```python
from build123d import *

# Parameters (mm, degrees)
BOSS_EXTRUDE1_DEPTH = 1.524
CUT_EXTRUDE1_DEPTH  = 1.524


with BuildPart() as part:
    # Sketch1 → Boss-Extrude1 (new body)
    with BuildSketch(Plane.XY):
        with BuildLine():
            Line((-65.62844389, -1.524), (-63.025670989, -1.524))
            Line((-63.025670989, -1.524), (-63.822514801, -3.597982164))
            Line((-63.822514801, -3.597982164), (-66.364740688, -5.02874479))
            Line((-66.364740688, -5.02874479), (-72.970412181, -5.02874479))
            ThreePointArc((-72.970412181, -5.02874479), (-73.780479042, -4.88253576), (-74.589728748, -4.731869528))
            Line((-74.589728748, -4.731869528), (-75.073084302, -7.372952412))
            Line((-75.073084302, -7.372952412), (-75.51502387, -4.553940069))
            ThreePointArc((-75.51502387, -4.553940069), (-79.267617574, -3.769993691), (-82.998880802, -2.890103837))
            Line((-82.998880802, -2.890103837), (-83.662208167, -4.580640418))
            Line((-83.662208167, -4.580640418), (-83.9742265, -2.643374593))
            ThreePointArc((-83.9742265, -2.643374593), (-87.594512539, -1.666053196), (-91.189152721, -0.598256357))
            Line((-91.189152721, -0.598256357), (-91.929187087, -1.873078309))
            Line((-91.929187087, -1.873078309), (-92.192549363, -0.282576404))
            ThreePointArc((-92.192549363, -0.282576404), (-94.43829357, 0.452244536), (-96.672145794, 1.2224608))
            ThreePointArc((-96.672145794, 1.2224608), (-98.79856677, 2.920982901), (-100.989304929, 4.535699537))
            Line((-100.989304929, 4.535699537), (-102.141504416, 2.851715672))
            Line((-102.141504416, 2.851715672), (-101.830844258, 5.121924515))
            ThreePointArc((-101.830844258, 5.121924515), (-105.503835902, 7.476274523), (-109.316148256, 9.597619873))
            Line((-109.316148256, 9.597619873), (-110.95226101, 7.891468444))
            Line((-110.95226101, 7.891468444), (-110.319639872, 10.105642428))
            ThreePointArc((-110.319639872, 10.105642428), (-116.815196671, 12.929470472), (-123.562513889, 15.083530197))
            ThreePointArc((-123.562513889, 15.083530197), (-123.779823463, 15.177511529), (-123.959746364, 15.331406595))
            ThreePointArc((-123.959746364, 15.331406595), (-123.949496649, 18.088692586), (-121.216404531, 18.453300008))
            ThreePointArc((-121.216404531, 18.453300008), (-119.99831308, 17.594979685), (-118.73086738, 16.811371391))
            Line((-118.73086738, 16.811371391), (-117.11063531, 18.184449417))
            Line((-117.11063531, 18.184449417), (-117.859531811, 16.331247904))
            ThreePointArc((-117.859531811, 16.331247904), (-113.341616748, 14.499894981), (-108.552725398, 13.587793188))
            ThreePointArc((-108.552725398, 13.587793188), (-107.803028846, 13.376700844), (-107.057015293, 13.152940531))
            Line((-107.057015293, 13.152940531), (-106.609325514, 15.13772615))
            Line((-106.609325514, 15.13772615), (-106.122626057, 12.853069881))
            ThreePointArc((-106.122626057, 12.853069881), (-103.421109493, 11.859213859), (-100.787074077, 10.698266414))
            Line((-100.787074077, 10.698266414), (-99.448684771, 12.381094003))
            Line((-99.448684771, 12.381094003), (-100.023702083, 10.324148845))
            ThreePointArc((-100.023702083, 10.324148845), (-96.831167643, 8.560951785), (-93.788416789, 6.550278449))
            Line((-93.788416789, 6.550278449), (-92.677002467, 8.368956431))
            Line((-92.677002467, 8.368956431), (-92.959454339, 5.939754488))
            ThreePointArc((-92.959454339, 5.939754488), (-91.397772197, 4.708540381), (-89.890787426, 3.410951775))
            ThreePointArc((-89.890787426, 3.410951775), (-84.591869737, 0.643036614), (-78.809267625, 2.160071819))
            ThreePointArc((-78.809267625, 2.160071819), (-77.644578081, 2.700645179), (-76.424081928, 3.09953167))
            Line((-76.424081928, 3.09953167), (-76.558408494, 5.228958142))
            Line((-76.558408494, 5.228958142), (-75.149258413, 3.353285973))
            ThreePointArc((-75.149258413, 3.353285973), (-73.933139466, 3.450839152), (-72.713766302, 3.410951775))
            Line((-72.713766302, 3.410951775), (-66.233949818, 3.410951775))
            Line((-66.233949818, 3.410951775), (-63.424092895, 1.94149826))
            Line((-63.424092895, 1.94149826), (-63.025670989, 0))
            Line((-63.025670989, 0), (-65.62844389, 0))
            Line((-65.62844389, 0), (-65.62844389, -1.524))
        make_face()
    extrude(amount=BOSS_EXTRUDE1_DEPTH)

    # Sketch2 → Cut-Extrude1 (cut)
    with BuildSketch(Plane.XY.offset(1.524)):
        Polygon((-126.267748699, 16.679917712), (-121.799652461, 15.482694933), (-121.405212236, 16.954765892), (-125.873308475, 18.151988671), align=None)
    extrude(amount=-CUT_EXTRUDE1_DEPTH, mode=Mode.SUBTRACT)


solid = part.part
```
For this review, take the finished solid that the model builds, in its own axes (mm). A direction names the side the tool comes from. Round coordinates to 2 decimals unless told otherwise and drop trailing zeros. Write each loop counter-clockwise with the first axis right and the second up, starting at its lowest first coordinate (ties: lowest second). Pieces come first, ordered by that corner, then holes. Notation, with made-up numbers: (48.25, 28.25) - (52.25, 28.25) arc R15 ccw to (52.25, 54.25) - close; hole circle Ø9 at (30, -16.5). An arc over 180 degrees is marked (long way). Answer as a JSON object with one key per item and string values.
1. We need section C-C on x = -114.5. Give the boundary of the cut face in (y, z).
Response values:
{"outline": "(12.01, 0) - (14.87, 0) - (14.87, 1.52) - (12.01, 1.52) - close"}
2. We need section A-A on y = 4. Give the boundary of the cut face in (x, z), then the cut area to 3 significant figures.
Response values:
{"outline": "(-101.98, 0) - (-101.36, 0) - (-101.36, 1.52) - (-101.98, 1.52) - close; (-100.24, 0) - (-90.56, 0) - (-90.56, 1.52) - (-100.24, 1.52) - close; (-76.48, 0) - (-75.64, 0) - (-75.64, 1.52) - (-76.48, 1.52) - close", "area": "17.0 mm2"}
3. To check wall thickness, follow line 1 along X through (y, z) = (9.5, 0.35); line 2 along X through (y, z) = (9.25, 1.25); line 3 along Y through (x, z) = (-82, 0.8). State the ranges of each line that lie inside material, in increasing order.
Response values:
{"line 1": "x = -110.49 to -109.41, -109.13 to -98.46", "line 2": "x = -110.56 to -109.65, -108.65 to -98.01", "line 3": "y = -3.14 to 0.76"}
4. Tool access review of faces 1 (the face through (-110.64, 8.98, 0.75)), 2 (the face through (-121.605, 16.208, 0.773)), 3 (the face through (-117.48, 17.27, 0.75)), 4 (the face through (-73.769, -4.885, 0.751)), 5 (the face through (-103.458, 11.874, 0.751)): name each direction out of +Z, -Z, +X, -X, +Y, -Y from which nothing blocks a thin tool from reaching the whole face with its end or side.
Response values:
{"face 1": "+Z, -Z, -X", "face 2": "+Z, -Z", "face 3": "+Z, -Z, +X", "face 4": "+Z, -Z, -Y", "face 5": "+Z, -Z, +Y"}
5. We need section B-B on x = -68. Give the boundary of the cut face in (y, z), then the cut area to 3 significant figures.
Response values:
{"outline": "(-5.03, 0) - (3.41, 0) - (3.41, 1.52) - (-5.03, 1.52) - close", "area": "12.9 mm2"}
6. Draft analysis for pull direction X (two halves, no side actions). For faces 6 (the face through (-106.37, 14.01, 0.75)), 7 (the face through (-122.791, 17.326, 0.773)), 8 (the face through (-79.22, -3.78, 0.75)), state which applies: +X half, -X half, draft (parallel to the pull), parting line (faces both ways), or undercut.
Response values:
{"face 6": "+X half", "face 7": "-X half", "face 8": "undercut"}
7. For pin 1 Ø0.8 at (x, z) = (-64, 1) entering from +Y; pin 2 Ø0.8 at (x, z) = (-64, 0.5) entering from -Y; pin 3 Ø0.8 at (y, z) = (-1, 1) entering from +X; pin 4 Ø1 at (x, y) = (-86.5, 1) entering from -Z, all flat-tipped, find the tip position at first contact; note any pin that passes through.
Response values:
{"pin 1": "stops at y = 2.45", "pin 2": "stops at y = -3.92", "pin 3": "stops at x = -65.63", "pin 4": "stops at z = 0"}
